Design review of the part built by this model. Coordinates are the model's own, in mm. Give positions to 0.01 mm unless a question says otherwise; leave off trailing zeros. Write each loop counter-clockwise with the first axis right and the second up, starting at its lowest first coordinate (ties: lowest second). Pieces come first, ordered by that corner, then holes. Notation, with made-up numbers: (-17.5, -6) - (18.5, -6) arc R18 cw to (18.5, 21) - close; hole circle Ø9 at (13, -15). An arc over 180 degrees is marked (long way). Write each question's results on one line, items separated by ' | '. Start each with the question number.
from build123d import *

# Parameters (mm, degrees)
BOSS_EXTRUDE1_DEPTH = 101.6


with BuildPart() as part:
    # Sketch1 → Boss-Extrude1 (new body, symmetric)
    with BuildSketch(Plane(origin=(0, 0, 0), x_dir=(0, 0, -1), z_dir=(1, 0, 0))):
        with BuildLine():
            Line((49.373646209, 66.02166065), (-1.426353791, 66.02166065))
            Line((-1.426353791, 66.02166065), (-1.426353791, -60.97833935))
            Line((-1.426353791, -60.97833935), (49.373646209, -60.97833935))
            ThreePointArc((49.373646209, -60.97833935), (71.824286512, -51.678979653), (81.123646209, -29.22833935))
            Line((81.123646209, -29.22833935), (81.123646209, 34.27166065))
            ThreePointArc((81.123646209, 34.27166065), (71.824286512, 56.722300952), (49.373646209, 66.02166065))
        make_face()
    extrude(amount=BOSS_EXTRUDE1_DEPTH, both=True)


solid = part.part
Q1. Insertion check: P1, Ø12, axis at x = 14.5, z = -61.5, coming from the -Y side; P2, Ø4, axis at x = -42.5, y = 42.5, coming from the -Z side. Each pin has a flat end and moves straight along its axis. Give the tip position at first contact, or say it passes through.
Q2. Add section C-C on z = -74. State the section outline as (x, y) points.
Q3. For line 1 along Z through (x, y) = (46, -30.5); line 2 along Z through (x, y) = (0.5, -54); line 3 along Y through (x, z) = (11, -67.5), list the stretches that pass through material, from the lowest coordinate up. Write a range as [from, to].
Q4. Add section B-B on y = -43. State the section outline as (x, z) points, plus the area to 3 significant figures.
Q5. Add section A-A on x = 28.5. State the section outline as (y, z) points.
Result:
1) P1: stops at y = -60.38 | P2: stops at z = -80.51
2) outline: (-101.6, -49.27) - (101.6, -49.27) - (101.6, 54.31) - (-101.6, 54.31) - close
3) line 1: z = [-81.1, 1.43] | line 2: z = [-69.23, 1.43] | line 3: y = [-55.3, 60.34]
4) outline: (-101.6, -77.98) - (101.6, -77.98) - (101.6, 1.43) - (-101.6, 1.43) - close | area: 16,100 mm²
5) outline: (-60.98, -49.37) arc R31.75 ccw to (-29.23, -81.12) - (34.27, -81.12) arc R31.75 ccw to (66.02, -49.37) - (66.02, 1.43) - (-60.98, 1.43) - close
